from build123d import *

# Parameters (mm, degrees)
FILLET1_R = 0.1


with BuildPart() as part:
    # Sketch1 → Revolve1 (revolve)
    with BuildSketch(Plane.XY):
        Polygon((0, 0), (0, 4), (1, 4), (1, 2.075), (16, 2.075), (16, 1.5), (17, 1.5), (17, 2.075), (18, 2.075), (18, 0), align=None)
    revolve(axis=Axis((-1.619660583, 0, 0), (1, 0, 0)))

    # Fillet1
    fillet1_edges = [part.edges().sort_by_distance(p)[0] for p in [
        (1, -4, 0),
        (0, -4, 0),
        (18, -2.075, 0),
    ]]
    fillet(fillet1_edges, radius=FILLET1_R)


solid = part.part
The listing builds one solid part. Answer for the finished solid, in the listing's coordinates (mm). A direction names the side the tool comes from. Give positions to 0.01 mm unless a question says otherwise; leave off trailing zeros. Write each loop counter-clockwise with the first axis right and the second up, starting at its lowest first coordinate (ties: lowest second). Pieces come first, ordered by that corner, then holes. Notation, with made-up numbers: (10.25, -26.75) -> (55.25, -26.75) arc R36 cw to (55.25, 10.25) -> close; hole circle Ø10 at (-25.75, 23.25). An arc over 180 degrees is marked (long way). One line per question, with ' | ' between items. Start each with the question number.
1. Section C-C (x = 14.25) is taken. Determine the outline of the cut face in (y, z) (3 decimals).
2. For a pull along X with two mould halves and no side action, classify faces 1 (the cylindrical face through (0.506, -0.867, -3.905)), 2 (the cylindrical face through (16.51, -1.5, 0.07)), 3 (the flat face through (0, 0, 0)), 4 (the flat face through (1, 2, -2)) as pulls with the +X half, pulls with the -X half, needs draft (parallel to the pull), parting line crosses it, or undercut.
3. Find the intervals of material crossed by probe 1 along X at (y, z) = (-1.5, 0.5); probe 2 along X at (y, z) = (-3, -1.5); probe 3 along Z at (x, y) = (3, 0) (3 decimals), in increasing order.
4. Section A-A (y = 0) is taken. Determine the outline of the cut face in (x, z) (3 decimals), plus the area to 3 significant figures.
5. For faces 5 (the flat face through (18, 0, 0)), 6 (the cylindrical face through (17.456, -0.45, -2.026)), determine the directions among +Z, -Z, +X, -X, +Y, -Y from which every point of the face is accessible in a straight line to the end or side of a thin tool.
6. Given pin 1 Ø1.2 at (y, z) = (1, 1) entering from -X; pin 2 Ø1 at (x, y) = (3.5, -0.5) entering from +Z (3 decimals), each flat-ended and moving along its own axis, determine where each tip first touches the part or whether it passes through.
Response values:
1) outline: circle Ø4.15 at (0, 0)
2) face 1: needs draft | face 2: undercut | face 3: pulls with the -X half | face 4: pulls with the +X half
3) probe 1: 0 to 16, 17 to 18 | probe 2: 0 to 1 | probe 3: -2.075 to 2.075
4) outline: (0, -3.9) arc R0.1 ccw to (0.1, -4) -> (0.9, -4) arc R0.1 ccw to (1, -3.9) -> (1, -2.075) -> (16, -2.075) -> (16, -1.5) -> (17, -1.5) -> (17, -2.075) -> (17.9, -2.075) arc R0.1 ccw to (18, -1.975) -> (18, 1.975) arc R0.1 ccw to (17.9, 2.075) -> (17, 2.075) -> (17, 1.5) -> (16, 1.5) -> (16, 2.075) -> (1, 2.075) -> (1, 3.9) arc R0.1 ccw to (0.9, 4) -> (0.1, 4) arc R0.1 ccw to (0, 3.9) -> close | area: 77.4 mm2
5) face 5: +Z, -Z, +X, +Y, -Y | face 6: +X
6) pin 1: x = 0 | pin 2: z = 2.075
